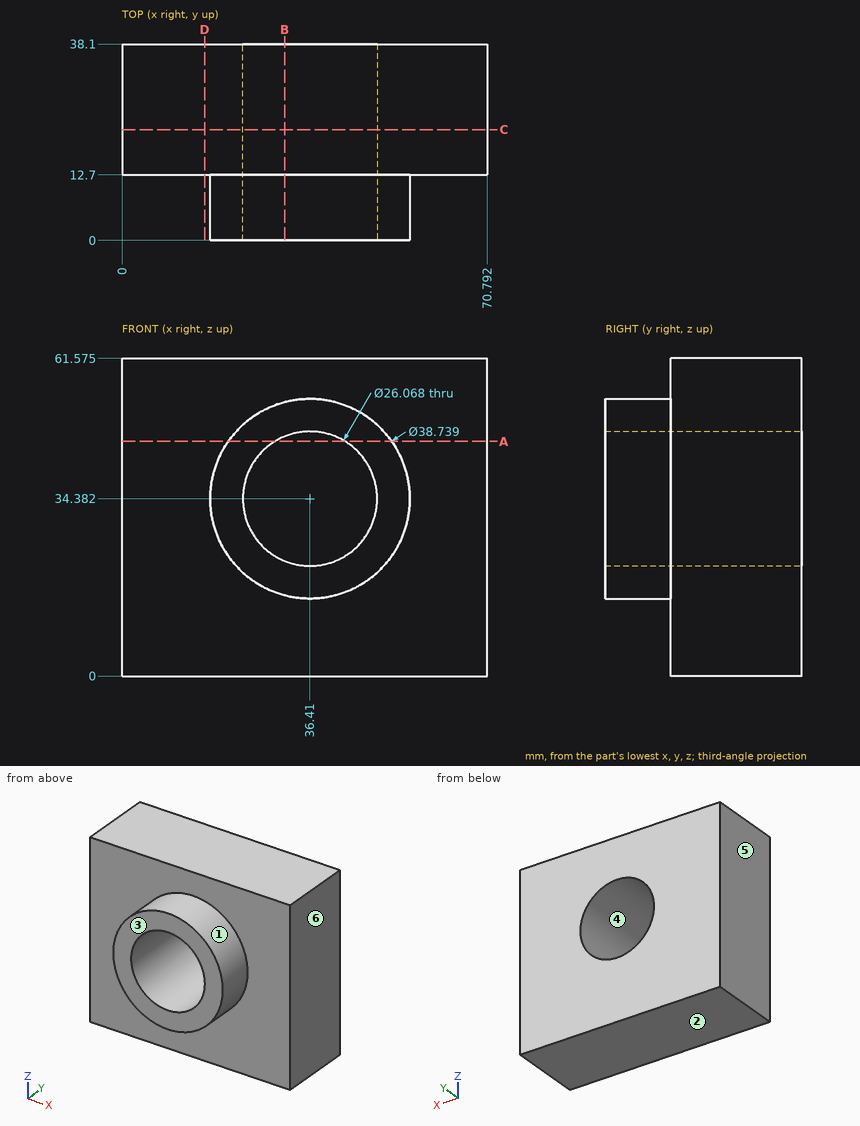
Could you check a few things on this drawing? It's one solid part, dimensions in mm from its lowest x, y, z. A direction names the side the tool comes from. Round coordinates to 2 decimals unless told otherwise and drop trailing zeros. Write each loop counter-clockwise with the first axis right and the second up, starting at its lowest first coordinate (ties: lowest second). Pieces come first, ordered by that corner, then holes. Notation, with made-up numbers: (5, 63.5) -> (9, 63.5) arc R14 cw to (9, 84.5) -> close; hole circle Ø3 at (-5.5, 15.25). An arc over 180 degrees is marked (long way). One line per item, written item: value.
1) If I drill on line 1 (Y direction, x = 16, z = 48); line 2 (Z direction, x = 38.5, y = 36) (1 decimal); line 3 (X direction, y = 27, z = 28) (1 decimal), over which ranges is the centre line in solid material (lowest first)? Write a range as [from, to].
Filled sheet:
line 1: y = [12.7, 38.1]
line 2: z = [0, 21.5], [47.2, 61.6]
line 3: x = [0, 25], [47.8, 70.8]
2) Suppose I cut it at A-A on z = 45.5. List the corners of the cut face in (x, y) for me.
Filled sheet:
outline: (0, 12.7) -> (20.55, 12.7) -> (20.55, 0) -> (29.61, 0) -> (29.61, 38.1) -> (0, 38.1) -> close; (43.21, 0) -> (52.27, 0) -> (52.27, 12.7) -> (70.79, 12.7) -> (70.79, 38.1) -> (43.21, 38.1) -> close
3) For the marked faces 1 and 2, which set-ups out of +Z, -Z, +X, -X, +Y, -Y let a thin tool reach every point of the face, with its end or its side?
Filled sheet:
face 1: -Y
face 2: -Z, +X, -X, +Y, -Y
4) I'm going to push flat-ended pins straight in: pin 1 Ø8 at (x, z) = (45, 43.5) entering from +Y; pin 2 Ø4 at (x, z) = (52.5, 17) entering from -Y; pin 3 Ø21 at (x, z) = (36.41, 34.38) entering from -Y; pin 4 Ø3 at (y, z) = (4, 38) entering from +X. Where does each tip first touch, or does it pass through?
Filled sheet:
pin 1: stops at y = 38.1
pin 2: stops at y = 12.7
pin 3: passes through
pin 4: stops at x = 55.66
5) Suppose I cut it at B-B on x = 31.5. List the corners of the cut face in (y, z) for me (1 decimal).
Filled sheet:
outline: (0, 15.6) -> (12.7, 15.6) -> (12.7, 0) -> (38.1, 0) -> (38.1, 22.3) -> (0, 22.3) -> close; (0, 46.5) -> (38.1, 46.5) -> (38.1, 61.6) -> (12.7, 61.6) -> (12.7, 53.1) -> (0, 53.1) -> close
6) Suppose I cut it at D-D on x = 16. List the corners of the cut face in (y, z) for me (1 decimal), plus the area to 3 significant figures.
Filled sheet:
outline: (12.7, 0) -> (38.1, 0) -> (38.1, 61.6) -> (12.7, 61.6) -> close
area: 1,560 mm2
7) Suppose I cut it at C-C on y = 21.5. List the corners of the cut face in (x, z) for me (1 decimal).
Filled sheet:
outline: (0, 0) -> (70.8, 0) -> (70.8, 61.6) -> (0, 61.6) -> close; hole circle Ø26.1 at (36.4, 34.4)
8) We'd pull the mould along X, two halves only. Please class the marked faces 3, 4, 5 and 6: released by +X, released by -X, zero draft, split by the parting line, or undercut.
Filled sheet:
face 3: zero draft
face 4: undercut
face 5: released by -X
face 6: released by +X
